Verification items for the finished model (mm, model axes). Face numbers are marked on the shaded views. A direction names the side the tool comes from. Give positions to 0.01 mm unless a question says otherwise; leave off trailing zeros. Write each loop counter-clockwise with the first axis right and the second up, starting at its lowest first coordinate (ties: lowest second). Pieces come first, ordered by that corner, then holes.
from build123d import *

# Parameters (mm, degrees)
HOLE_WIZARD_G1_8_1_D           = 8.8
HOLE_WIZARD_G1_8_1_CSINK_D     = 9.778
HOLE_WIZARD_G1_8_1_CSINK_ANGLE = 90
FILLET_1_R                     = 1
SKETCH_5_W                     = 32.896271037
SKETCH_5_H                     = 64.386050675
CUT_EXTRUDE_1_DEPTH            = 10
SKETCH_6_R                     = 4.4
EXTRUDE_1_DEPTH                = 5
FILLET_2_R                     = 0.5


with BuildPart() as part:
    # 草图1 → 旋转2 (revolve)
    with BuildSketch(Plane.XY, mode=Mode.PRIVATE) as revolve_2_sk:
        Polygon((-40.5, 0), (-41.5, 0), (-30, 8.651787717), (-42.5, 18.178475316), (-30, 30), (-30, 37), (-22.5, 37), (-22.5, 48.5), (-7, 48.5), (-7, 78.5), (0, 78.5), (0, 30), (-29, 30), (-41.5, 18.178475316), (-29, 8.651787717), align=None)
    revolve(revolve_2_sk.sketch.rotate(Axis((0, 0, 0), (0, 1, 0)), 270), axis=Axis((0, 0, 0), (0, 1, 0)))

    # G1/8 螺纹孔1 (through all)
    with Locations(Plane(origin=(0, 78.5, 0), x_dir=(1, 0, 0), z_dir=(0, 1, 0))):
        with Locations((0, 0)):
            CounterSinkHole(HOLE_WIZARD_G1_8_1_D / 2, HOLE_WIZARD_G1_8_1_CSINK_D / 2, counter_sink_angle=HOLE_WIZARD_G1_8_1_CSINK_ANGLE)

    # 圆角1
    fillet_1_edges = [part.edges().sort_by_distance(p)[0] for p in [
        (0, 78.5, 7),
    ]]
    fillet(fillet_1_edges, radius=FILLET_1_R)

    # 草图5 → 切除-拉伸1 (cut)
    with BuildSketch(Plane(origin=(0, 48.5, 0), x_dir=(1, 0, 0), z_dir=(0, 1, 0))):
        with Locations((-34.448135519, 0.195346028)):
            Rectangle(SKETCH_5_W, SKETCH_5_H)
        with Locations((34.448135519, 0.195346028)):
            Rectangle(SKETCH_5_W, SKETCH_5_H)
    extrude(amount=-CUT_EXTRUDE_1_DEPTH, mode=Mode.SUBTRACT)

    # 草图6 → 凸台-拉伸1 (add)
    with BuildSketch(Plane(origin=(0, 48.5, 0), x_dir=(1, 0, 0), z_dir=(0, 1, 0))):
        Polygon((0, 10.969655115), (-9.5, 5.484827557), (-9.5, -5.484827557), (0, -10.969655115), (9.5, -5.484827557), (9.5, 5.484827557), align=None)
        with Locations(Location((0, 0, 0), (0, 0, 270))):
            Circle(SKETCH_6_R, mode=Mode.SUBTRACT)
    extrude(amount=EXTRUDE_1_DEPTH)

    # 圆角2
    fillet_2_edges = [part.edges().sort_by_distance(p)[0] for p in [
        (9.5, 51, -5.484827557),
        (0, 51, -10.969655115),
        (-9.5, 51, -5.484827557),
        (-9.5, 51, 5.484827557),
        (0, 51, 10.969655115),
        (9.5, 51, 5.484827557),
    ]]
    fillet(fillet_2_edges, radius=FILLET_2_R)


solid = part.part
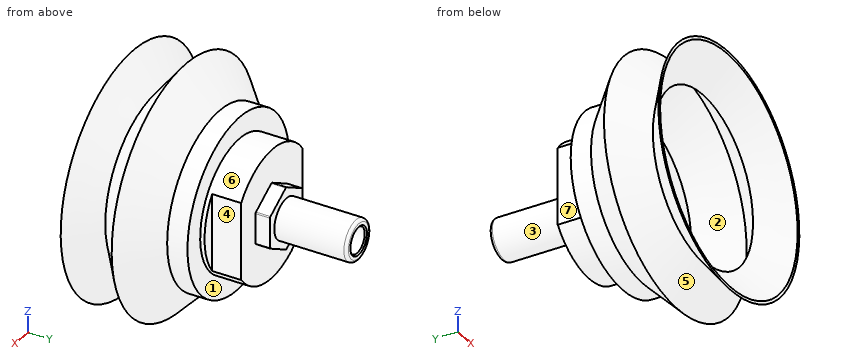
Item 1: Release check for a two-part mould opening along Z. For the marked faces 1, 2 and 3 record: released by +Z, released by -Z, zero draft, split by the parting line, or undercut.
Answer key:
face 1: zero draft
face 2: undercut
face 3: split by the parting line
Item 2: Scan lines: line 1 along Z through (x, y) = (0, 50); line 2 along Y through (x, z) = (-33, 21); line 3 along Y through (x, z) = (38.5, 13). Record each from-to range of solid material in increasing order.
Answer key:
line 1: z = -10.89 to -4.4, 4.4 to 10.89
line 2: y = 1.04 to 1.79, 15.6 to 16.36, 20.43 to 21.38
line 3: y = 0 to 0.65, 16.76 to 17.52, 19 to 19.94
Item 3: Set-up check for the marked faces 4, 5, 6 and 7: record each of +Z, -Z, +X, -X, +Y, -Y from which the full face is reachable in a straight line by a thin tool's end or side.
Answer key:
face 4: +Z, -Z, +X, +Y
face 5: none
face 6: +Y
face 7: +Z, -Z, -X, +Y
Item 4: Sectioned sample at B-B on x = 33. State how many separate pieces and enclosed holes the cut face has, then the cut area to 3 significant figures.
Answer key:
separate pieces: 2
enclosed holes: 1
area: 125 mm2
Item 5: Depth check by flat-ended pin: pin 1 (21 mm diameter, centred on x = 4, z = 0, fed in from +Y); pin 2 (2 mm diameter, centred on x = 20.5, z = -4.5, fed in from +Y); pin 3 (6 mm diameter, centred on x = 2.5, y = 9.5, fed in from -Z); pin 4 (8 mm diameter, centred on y = 27.5, z = 17.5, fed in from -X). Enter the tip coordinate at first touch or a pass-through.
Answer key:
pin 1: stops at y = 78.5
pin 2: stops at y = 38.5
pin 3: stops at z = -34.97
pin 4: stops at x = -32.88
Item 6: Sectioned sample at D-D on y = 60. Record the cut outline in (x, z).
Answer key:
outline: circle Ø14 at (0, 0); hole circle Ø8.8 at (0, 0)
Item 7: Sectioned sample at A-A on y = 43. Record the cut outline in (x, z), then the cut area to 3 significant figures.
Answer key:
outline: (-18, -13.5) arc R22.5 ccw to (18, -13.5) - (18, 13.5) arc R22.5 ccw to (-18, 13.5) - close; hole circle Ø8.8 at (0, 0)
area: 1,360 mm2
